```python
from build123d import *

# Parameters (mm, degrees)
F0_R     = 2.5
F0_R_2   = 1.85
F1_DEPTH = 4.5
F2_R     = 0.5
F3_DEPTH = 2.3


with BuildPart() as f1:
    # F0 (on Top) → F1 (new body)
    with BuildSketch(Plane.XY):
        Circle(F0_R)
        Circle(F0_R_2, mode=Mode.SUBTRACT)
        Circle(F0_R_2)
    extrude(amount=F1_DEPTH)

    # F2
    f2_edges = [f1.edges().sort_by_distance(p)[0] for p in [
        (-2.5, 0, 4.5),
    ]]
    fillet(f2_edges, radius=F2_R)

    # F0 (on Top) → F3 (cut)
    with BuildSketch(Plane.XY):
        Circle(F0_R_2)
    extrude(amount=F3_DEPTH, mode=Mode.SUBTRACT)


solid = f1.part
```
Input: part model. Units: mm. Frame: model coordinates. A direction names the side the tool comes from. Round coordinates to 2 decimals unless told otherwise and drop trailing zeros. Loops run counter-clockwise (first coordinate to the right, second up) from the corner with the lowest first, then second, coordinate; pieces in that order, holes last. Notation, with made-up numbers: (66.25, -2) -> (85.25, -2) arc R17 ccw to (85.25, 6) -> close; hole circle Ø7 at (41, 62). An arc over 180 degrees is marked (long way). Use one line per item in the form item = value. Start each with the question number.
Item 1: Material intervals for L1, parallel to Y at x = 0, z = 1.1; L2, parallel to Z at x = 0.95, y = -0.05; L3, parallel to Y at x = 1.5, z = 2, sorted ascending. Write a range as from..to.
Item 2: Contact query for flat-ended pins moving along their axis: pin 1 Ø3 at (x, y) = (0, 0) entering from -Z; pin 2 Ø1.5 at (x, z) = (-1.5, 2) entering from +Y; pin 3 Ø1 at (y, z) = (-1, 1) entering from -X. Output: stop coordinate, or through.
Item 3: Mould query, pull axis Y, two halves, no side actions, for faces 3 (the face through (-2, 1, 0)), 4 (the face through (-0.401, -1.806, 1.134)), 5 (the face through (-0.54, -2.44, 1.97)). Classes: pulls with the +Y half, pulls with the -Y half, needs draft (parallel to the pull), parting line crosses it, or undercut.
Item 4: Section query D-D on z = 2.7. Return the cut outline in (x, y), then the cut area to 3 significant figures.
Item 5: Set-up query: faces 1 (the face through (0, 0, 2.3)), 2 (the face through (0, 0, 4.5)). Return all of +Z, -Z, +X, -X, +Y, -Y with unobstructed straight access to the full face (end or side cutting, diameter ignored); none if empty.
Item 6: Section query A-A on y = 0. Return the cut outline in (x, z), then the cut area to 3 significant figures.
Item 7: Section query C-C on z = 0.4. Return the cut outline in (x, y), then the cut area to 3 significant figures.
Ans:
q1.L1 = -2.5..-1.85, 1.85..2.5
q1.L2 = 2.3..4.5
q1.L3 = -2..-1.08, 1.08..2
q2.pin_1 = 2.3
q2.pin_2 = 2.38
q2.pin_3 = -2.45
q3.face_3 = needs draft
q3.face_4 = undercut
q3.face_5 = parting line crosses it
q4.outline = circle Ø5 at (0, 0)
q4.area = 19.6 mm^2
q5.face_1 = -Z
q5.face_2 = +Z, +X, -X, +Y, -Y
q6.outline = (-2.5, 0) -> (-1.85, 0) -> (-1.85, 2.3) -> (1.85, 2.3) -> (1.85, 0) -> (2.5, 0) -> (2.5, 4) arc R0.5 ccw to (2, 4.5) -> (-2, 4.5) arc R0.5 ccw to (-2.5, 4) -> close
q6.area = 13.9 mm^2
q7.outline = circle Ø5 at (0, 0); hole circle Ø3.7 at (0, 0)
q7.area = 8.88 mm^2
